```python
from build123d import *

# Parameters (mm, degrees)
ESTRUSIONE_ESTRUSIONE1_DEPTH = 5
RACCORDO1_R                  = 0.25
SCHIZZO7_R                   = 2
ESTRUSIONE_ESTRUSIONE3_DEPTH = 16
SMUSSO1_SIZE                 = 0.25


with BuildPart() as part:
    # Schizzo1 → Estrusione-Estrusione1 (new body)
    with BuildSketch(Plane.XY):
        Polygon((3.7, 0), (-3.7, 0), (-6, 2.3), (-6, 3.3), (-3, 3.3), (-3, 5), (3, 5), (3, 3.3), (6, 3.3), (6, 2.3), align=None)
    extrude(amount=ESTRUSIONE_ESTRUSIONE1_DEPTH)

    # Raccordo1
    raccordo1_edges = [part.edges().sort_by_distance(p)[0] for p in [
        (-6, 2.8, 0),
        (-4.5, 3.3, 0),
        (-3, 4.15, 0),
        (0, 5, 0),
        (3, 4.15, 0),
        (4.5, 3.3, 0),
        (6, 2.8, 0),
        (4.85, 1.15, 5),
        (4.85, 1.15, 0),
        (0, 0, 0),
        (-4.85, 1.15, 0),
        (6, 2.8, 5),
        (-6, 2.3, 2.5),
        (-6, 3.3, 2.5),
        (-3, 3.3, 2.5),
        (-3, 5, 2.5),
        (3, 5, 2.5),
        (3, 3.3, 2.5),
        (-3.7, 0, 2.5),
        (4.5, 3.3, 5),
        (3, 4.15, 5),
        (0, 5, 5),
        (-3, 4.15, 5),
        (-4.5, 3.3, 5),
        (-6, 2.8, 5),
        (-4.85, 1.15, 5),
        (0, 0, 5),
    ]]
    fillet(raccordo1_edges, radius=RACCORDO1_R)

    # Schizzo7 → Estrusione-Estrusione3 (add)
    with BuildSketch(Plane(origin=(0, 5, 0), x_dir=(1, 0, 0), z_dir=(0, 1, 0))):
        with Locations((0, -2.5)):
            Circle(SCHIZZO7_R)
    extrude(amount=ESTRUSIONE_ESTRUSIONE3_DEPTH)

    # Smusso1
    smusso1_edges = [part.edges().sort_by_distance(p)[0] for p in [
        (-2, 21, 2.5),
    ]]
    chamfer(smusso1_edges, length=SMUSSO1_SIZE)

    # Schizzo8 → Rivoluzione2 (revolve)
    with BuildSketch(Plane.XY.offset(1.25)):
        Polygon((-4.5, 3.3), (-4.5, 3.55), (-4.75, 3.3), align=None)
    rivoluzione2 = revolve(axis=Axis((-4.5, 3.3, 1.25), (0, 1, 0)))

    # Specchia3: Rivoluzione2 across plane
    add(rivoluzione2.mirror(Plane(origin=(0, 0, 0), x_dir=(0, 0, 1), z_dir=(1, 0, 0))))

    # Specchia4: Rivoluzione2 across plane
    add(rivoluzione2.mirror(Plane.XY.offset(2.5)))

    # Specchia4 copy 1 sketch → Specchia4 copy 1 (revolve)
    with BuildSketch(Plane(origin=(0, 0, 3.75), x_dir=(-1, 0, 0), z_dir=(0, 0, -1))):
        Polygon((-4.5, 3.3), (-4.5, 3.55), (-4.75, 3.3), align=None)
    revolve(axis=Axis((4.5, 3.3, 3.75), (0, 1, 0)))


solid = part.part
```
Could you check a few things on this model? Use its own coordinates, in mm. A direction names the side the tool comes from. Give positions to 0.01 mm unless a question says otherwise; leave off trailing zeros. Loops run counter-clockwise (first coordinate to the right, second up) from the corner with the lowest first, then second, coordinate; pieces in that order, holes last. Notation, with made-up numbers: (40.25, 6) -> (77.25, 6) arc R32 ccw to (77.25, 43) -> close; hole circle Ø6 at (35.5, -20.75). An arc over 180 degrees is marked (long way). Put each result on its own line as item: value.
(1) Imagine slicing it at D-D on y = 9.25. Write out the boundary of the cut face in (x, z).
Computed:
outline: circle Ø4 at (0, 2.5)
(2) Imagine slicing it at B-B on y = 4. Write out the boundary of the cut face in (x, z), plus the area to 3 significant figures.
Computed:
outline: (-3, 0.25) arc R0.25 ccw to (-2.75, 0) -> (2.75, 0) arc R0.25 ccw to (3, 0.25) -> (3, 4.75) arc R0.25 ccw to (2.75, 5) -> (-2.75, 5) arc R0.25 ccw to (-3, 4.75) -> close
area: 29.9 mm^2
(3) For faces 1 (the face through (3, 4, 2)), 2 (the face through (-0.434, 12.765, 4.452)), 3 (the face through (-3, 4, 2)), which set-ups out of +Z, -Z, +X, -X, +Y, -Y let a thin tool reach every point of the face, with its end or its side?
Computed:
face 1: +Z, -Z, +X, +Y
face 2: +Y
face 3: +Z, -Z, -X, +Y
(4) Please list where these lines run through material, in increasing order: probe 1 along X at (y, z) = (4.75, 4.4); probe 2 along X at (y, z) = (5.75, 2.5); probe 3 along Y at (x, z) = (2.25, 2.05). Write a range as [from, to].
Computed:
probe 1: [-3, 3]
probe 2: [-2, 2]
probe 3: [0, 5]
(5) Imagine slicing it at A-A on z = 2.5. Write out the boundary of the cut face in (x, y).
Computed:
outline: (-6, 2.4) arc R0.25 ccw to (-5.93, 2.23) -> (-3.77, 0.07) arc R0.25 ccw to (-3.6, 0) -> (3.7, 0) -> (6, 2.3) -> (6, 3.3) -> (3.25, 3.3) arc R0.25 cw to (3, 3.55) -> (3, 4.75) arc R0.25 ccw to (2.75, 5) -> (2, 5) -> (2, 20.75) -> (1.75, 21) -> (-1.75, 21) -> (-2, 20.75) -> (-2, 5) -> (-2.75, 5) arc R0.25 ccw to (-3, 4.75) -> (-3, 3.55) arc R0.25 cw to (-3.25, 3.3) -> (-5.75, 3.3) arc R0.25 ccw to (-6, 3.05) -> close
(6) Imagine slicing it at C-C on x = 0. Write out the boundary of the cut face in (y, z).
Computed:
outline: (0, 0.25) arc R0.25 ccw to (0.25, 0) -> (4.75, 0) arc R0.25 ccw to (5, 0.25) -> (5, 0.5) -> (20.75, 0.5) -> (21, 0.75) -> (21, 4.25) -> (20.75, 4.5) -> (5, 4.5) -> (5, 4.75) arc R0.25 ccw to (4.75, 5) -> (0.25, 5) arc R0.25 ccw to (0, 4.75) -> close
(7) I'm going to push flat-ended pins straight in: pin 1 Ø1.4 at (x, z) = (5, 2.5) entering from +Y; pin 2 Ø1.5 at (y, z) = (11, 4) entering from -X; pin 3 Ø1 at (y, z) = (4, 2.5) entering from +X. Where does each tip first touch, or does it pass through?
Computed:
pin 1: y = 3.3
pin 2: x = -1.85
pin 3: x = 3.01
